Can you work these out from the drawing? Everything is in mm from the part's minimum corner. A direction names the side the tool comes from. Give positions to 0.01 mm unless a question says otherwise; leave off trailing zeros. Order: outer loops, then holes, each group sorted by start corner. A loop starts at its lowest first (then second) coordinate and runs counter-clockwise, first axis right, second up. Notation, with made-up numbers: M 33.5,57.25 L 76.5,57.25 A28 ccw 76.5,95.25 Z; hole C -37,-17 d6. An arc over 180 degrees is marked long. Answer as a JSON object with one key per item and string values.
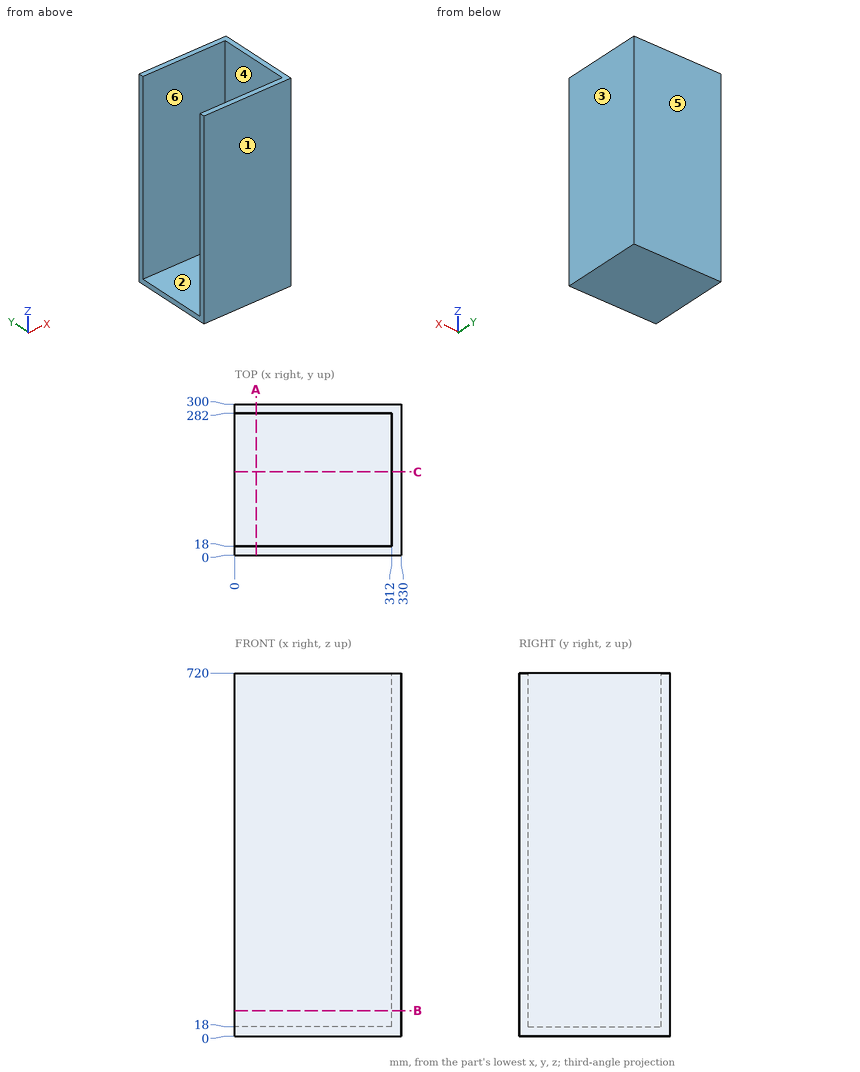
1) I need wall thicknesses on L1, parallel to Y at x = 54.5, z = 411; L2, parallel to Z at x = 188, y = 184.5; L3, parallel to X at y = 257.5, z = 261. Which ranges of each line are inside material? Lowest first, please.
Results found:
{"L1": "y = 0 to 18, 282 to 300", "L2": "z = 0 to 18", "L3": "x = 312 to 330"}
2) For the marked faces 1 and 2, which set-ups out of +Z, -Z, +X, -X, +Y, -Y let a thin tool reach every point of the face, with its end or its side?
Results found:
{"face 1": "+Z, -Z, +X, -X, -Y", "face 2": "+Z, -X"}
3) I want a section at C-C on y = 165.5. Write out the boundary of the cut face in (x, z).
Results found:
{"outline": "M 0,0 L 330,0 L 330,720 L 312,720 L 312,18 L 0,18 Z"}
4) Thinking about a two-plate mould opening in Y: for the marked faces 3, 4, 5 and 6, which applies, pulls with the +Y half, pulls with the -Y half, needs draft (parallel to the pull), parting line crosses it, or undercut?
Results found:
{"face 3": "needs draft", "face 4": "undercut", "face 5": "pulls with the +Y half", "face 6": "undercut"}
5) I want a section at A-A on x = 42.5. Write out the boundary of the cut face in (y, z), and give its area (3 significant figures).
Results found:
{"outline": "M 0,0 L 300,0 L 300,720 L 282,720 L 282,18 L 18,18 L 18,720 L 0,720 Z", "area": "30,700 mm²"}
6) I want a section at B-B on z = 50.5. Write out the boundary of the cut face in (x, y), and give its area (3 significant figures).
Results found:
{"outline": "M 0,0 L 330,0 L 330,300 L 0,300 L 0,282 L 312,282 L 312,18 L 0,18 Z", "area": "16,600 mm²"}
7) I'm going to push a flat-ended pin straight in: pin 1 Ø1 at (y, z) = (198.5, 443.5) entering from -X. Where does the tip first touch, or does it pass through?
Results found:
{"pin 1": "stops at x = 312"}
